Build history of the part. All positions in model axes, mm. A direction names the side the tool comes from. Round coordinates to 2 decimals unless told otherwise and drop trailing zeros. Write each loop counter-clockwise with the first axis right and the second up, starting at its lowest first coordinate (ties: lowest second). Pieces come first, ordered by that corner, then holes.
Item 1: Band-saw the part on B-B, the plane y = 1. Write the cut outline in (x, z).
Item 2: Band-saw the part on C-C, the plane z = -3.25. Write the cut outline in (x, y), then the cut area to 3 significant figures.
Item 3: 3-axis set-ups, long thin cutter, end or side, ignore diameter. For faces 1 (the flat face through (0, -7, 0)), 2 (the flat face through (0, 5, 0)), 3 (the cylindrical face through (-0.05, 7.23, -5.23)), 4 (the flat face through (0, 5, -8)), 5 (the cylindrical face through (0.369, -5.747, -2.827)): which of +Z, -Z, +X, -X, +Y, -Y reach the whole face in a straight line?
Item 4: Drop flat-ended pins along their axis: pin 1 Ø2.5 at (x, z) = (0, -4.5) entering from -Y; pin 2 Ø3.5 at (x, z) = (-7.5, 2) entering from +Y; pin 3 Ø2.5 at (x, y) = (-1.5, 3.5) entering from +Z; pin 4 Ø5 at (x, y) = (0, 0) entering from +Z. Give the stop position or say it passes through.
Item 5: Band-saw the part on A-A, the plane x = 0. Write the cut outline in (y, z).
Item 6: Band-saw the part on D-D, the plane x = -3.5. Write the cut outline in (y, z), then the cut area to 3 significant figures.
Item 7: Mould opens along Y. For faces 6 (the flat face through (0, -7, 3)), 7 (the cylindrical face through (0, -4, -4)), 8 (the cylindrical face through (1.63, 8.82, -3.94)) say: +Y half, -Y half, draft (parallel to the pull), parting line (faces both ways), or undercut.
Item 8: Wall check: probe 1 along Z at (x, y) = (0, -5.6); probe 2 along Z at (x, y) = (0, 7.95); probe 3 along Y at (x, z) = (0, -5.5). Give the ranges that are in metal, low to high.
Autodesk Inventor part; units mm, degrees
ref_plane "Work Plane1" through (0, 9, 0) normal (0, 1, 0) x (-1, 0, 0)
ref_plane "Work Plane2" through (0, 0, 0) normal (0, 1, 0) x (-1, 0, 0)
ref_plane "YZ Plane" through (0, 0, 0) normal (1, 0, 0) x (0, 1, 0)
sketch "Sketch1" plane through (0, 0, 0) normal (0, 0, 1) x (1, 0, 0)
  arc A0 (-14, 0) -> (14, 0) centre (0, 0) ccw
  line L0 (-14, 0) -> (14, 0)
  dimension "d0" = 28
extrude "Extrusion1" add sketch "Sketch1" along normal blind 3
sketch "Sketch2" plane through (0, 0, 0) normal (0, 0, -1) x (-1, 0, 0)
  circle A0 centre (0, 1.5) radius 7.5
  line L0 (-14, 0) -> (14, 0)
  point P0 (0, 0)
  point P1 (0, 0)
  dimension "d22" = 15
  dimension "d23" = 1.5
extrude "Extrusion2" add sketch "Sketch2" along normal blind 8
sketch "Sketch3" plane through (0, 0, -8) normal (0, 0, -1) x (-1, 0, 0)
  circle A0 centre (0, 1.5) radius 7.5
  point P0 (0, 0)
  point P1 (0, 0)
  point P2 (0, 0)
hole "Hole1" at (0, 0, -8) direction (0, 0, 1) diameter 8 depth 11
ref_plane "Work Plane1" through (0, 9, 0) normal (0, 1, 0) x (-1, 0, 0)
sketch "Sketch4" plane through (0, 9, 0) normal (0, 1, 0) x (-1, 0, 0)
  line L0 (-7.5, -8) -> (7.5, -8)
  line L1 (7.3485, 0) -> (-7.3485, 0)
  line L2 (7.3485, 0) -> (-7.3485, 0)
  line L3 (7.5, 0) -> (7.5, -8)
  line L4 (-7.5, 0) -> (-7.5, -8)
  point P0 (0, 0)
  point P1 (0, -4)
  point P2 (0, 0)
  point P3 (-7.5, -4)
hole "Hole2" at (0, 9, -4) direction (0, -1, 0) diameter 2.459 depth 3.5
ref_plane "Work Plane2" through (0, 0, 0) normal (0, 1, 0) x (-1, 0, 0)
mirror "Mirror1" about plane through (0, 0, 0) normal (0, 1, 0) of "Hole2"
properties part number "204"
Results:
1. outline: (-7.48, -8) - (-3.87, -8) - (-3.87, 0) - (-7.48, 0) - close; (3.87, -8) - (7.48, -8) - (7.48, 0) - (3.87, 0) - close
2. outline: (-0.97, -5.94) - (-0.97, -5.5) - (0.97, -5.5) - (0.97, -5.94) arc R7.5 ccw to (0.97, 8.94) - (0.97, 5.5) - (-0.97, 5.5) - (-0.97, 8.94) arc R7.5 ccw to start; hole circle Ø8 at (0, 0)
2. area: 119 mm2
3. face 1: -Z, -Y
3. face 2: +Z, +X, -X, +Y
3. face 3: +Y
3. face 4: -Z, +X, -X, +Y, -Y
3. face 5: -Y
4. pin 1: stops at y = -6
4. pin 2: stops at y = 0
4. pin 3: stops at z = 0
4. pin 4: passes through
5. outline: (-14, 0) - (-6, 0) - (-6, -2.77) - (-5.5, -2.77) - (-5.5, -5.23) - (-6, -5.23) - (-6, -8) - (-4, -8) - (-4, 3) - (-14, 3) - close; (4, -8) - (9, -8) - (9, -5.23) - (5.5, -5.23) - (5.5, -2.77) - (9, -2.77) - (9, 0) - (4, 0) - close
6. outline: (-13.56, 0) - (-5.13, 0) - (-5.13, -8) - (-1.94, -8) - (-1.94, 3) - (-13.56, 3) - close; (1.94, -8) - (8.13, -8) - (8.13, 0) - (1.94, 0) - close
6. area: 110 mm2
7. face 6: draft
7. face 7: undercut
7. face 8: parting line
8. probe 1: z = -8 to -5.23, -2.77 to 3
8. probe 2: z = -8 to -5.23, -2.77 to 0
8. probe 3: y = -6 to -4, 4 to 9
